Autodesk Inventor part; units mm, degrees
ref_plane "YZ Plane" through (0, 0, 0) normal (1, 0, 0) x (0, 1, 0)
ref_plane "XZ Plane" through (0, 0, 0) normal (0, 1, 0) x (-1, 0, 0)
ref_plane "XY Plane" through (0, 0, 0) normal (0, 0, 1) x (1, 0, 0)
sketch "Skizze1" plane through (0, 0, 0) normal (0, 0, 1) x (1, 0, 0)
  line L0 (-12.5, -12) -> (12.5, -12)
  line L1 (12.5, -12) -> (12.5, 12)
  line L2 (12.5, 12) -> (-12.5, 12)
  line L3 (-12.5, 12) -> (-12.5, -12)
  line L4 (-12.5, -12) -> (12.5, 12) construction
  line L5 (12.5, -12) -> (-12.5, 12) construction
  point P0 (0, 0)
  dimension "d0" = 25
  dimension "d1" = 24
extrude "Extrusion1" add sketch "Skizze1" along normal blind 1
sketch "Skizze2" plane through (0, 0, 1) normal (0, 0, 1) x (1, 0, 0)
  line L0 (-12.5, -12) -> (12.5, -12)
  line L1 (12.5, -12) -> (12.5, 12)
  line L2 (12.5, 12) -> (-12.5, 12)
  line L3 (-12.5, 12) -> (-12.5, -12)
  line L4 (12.5, 12) -> (-12.5, 12) construction
  line L5 (0, 12) -> (0, -12) construction
  line L6 (-12.5, -12) -> (12.5, -12) construction
  point P0 (0, 0)
  point P1 (-10.5, 10)
  point P2 (10.5, 10)
  point P3 (10.5, -3.5)
  point P4 (-10.5, -3.5)
  dimension "d4" = 2
  dimension "d5" = 2
  dimension "d6" = 8.5
  dimension "d7" = 2
hole "Bohrung1" at (-10.5, 10, 1) at (10.5, 10, 1) at (10.5, -3.5, 1) at (-10.5, -3.5, 1) direction (0, 0, -1) diameter 2.2 end through all
sketch "Skizze3" plane through (0, 0, 1) normal (0, 0, 1) x (1, 0, 0)
  circle A0 centre (10.5, -3.5) radius 1.1
  circle A1 centre (-10.5, 10) radius 1.1
  circle A2 centre (10.5, 10) radius 1.1
  circle A3 centre (-10.5, -3.5) radius 1.1
  line L0 (-12.5, -12) -> (12.5, -12)
  line L1 (12.5, -12) -> (12.5, 12)
  line L2 (12.5, 12) -> (-12.5, 12)
  line L3 (-12.5, 12) -> (-12.5, -12)
  line L4 (0, 12) -> (0, -12) construction
  point P0 (0, 0)
  point P1 (-9, 3)
  point P2 (9, 3)
  dimension "d16" = 9
  dimension "d17" = 18
hole "Bohrung2" at (-9, 3, 1) at (9, 3, 1) direction (0, 0, -1) diameter 1.82 end through all
properties part number "Waveshare Kamera PCB 24x25" material "Phenolharz"
Input: part model. Units: mm. Frame: model coordinates. Round coordinates to 2 decimals unless told otherwise and drop trailing zeros. Order: outer loops, then holes, each group sorted by start corner. A loop starts at its lowest first (then second) coordinate and runs counter-clockwise, first axis right, second up. Notation, with made-up numbers: (28, 25.5) - (65, 25.5) arc R30 ccw to (65, 56.5) - close; hole circle Ø7 at (69, -5). An arc over 180 degrees is marked (long way). Answer in a Markdown table with one row per item.
Item 1: Section query D-D (x = -10.5). Return the cut outline in (y, z).
Model answer:
| item | result |
|---|---|
| outline | (-12, 0) - (-4.6, 0) - (-4.6, 1) - (-12, 1) - close; (-2.4, 0) - (8.9, 0) - (8.9, 1) - (-2.4, 1) - close; (11.1, 0) - (12, 0) - (12, 1) - (11.1, 1) - close |
Item 2: Line query: line 1 (Y direction, x = -10.5, z = 0.55); line 2 (X direction, y = 10, z = 0.5); line 3 (X direction, y = -2.75, z = 0.7). Output: solid intervals per line, ascending.
Model answer:
| item | result |
|---|---|
| line 1 | y = -12 to -4.6, -2.4 to 8.9, 11.1 to 12 |
| line 2 | x = -12.5 to -11.6, -9.4 to 9.4, 11.6 to 12.5 |
| line 3 | x = -12.5 to -11.3, -9.7 to 9.7, 11.3 to 12.5 |
Item 3: Section query B-B (x = 9). Return the cut outline in (y, z).
Model answer:
| item | result |
|---|---|
| outline | (-12, 0) - (2.09, 0) - (2.09, 1) - (-12, 1) - close; (3.91, 0) - (12, 0) - (12, 1) - (3.91, 1) - close |
Item 4: Section query C-C (z = 0.8). Return the cut outline in (x, y).
Model answer:
| item | result |
|---|---|
| outline | (-12.5, -12) - (12.5, -12) - (12.5, 12) - (-12.5, 12) - close; hole circle Ø2.2 at (-10.5, -3.5); hole circle Ø2.2 at (-10.5, 10); hole circle Ø1.82 at (-9, 3); hole circle Ø1.82 at (9, 3); hole circle Ø2.2 at (10.5, -3.5); hole circle Ø2.2 at (10.5, 10) |
Item 5: Section query A-A (y = 3). Return the cut outline in (x, z).
Model answer:
| item | result |
|---|---|
| outline | (-12.5, 0) - (-9.91, 0) - (-9.91, 1) - (-12.5, 1) - close; (-8.09, 0) - (8.09, 0) - (8.09, 1) - (-8.09, 1) - close; (9.91, 0) - (12.5, 0) - (12.5, 1) - (9.91, 1) - close |
Item 6: Mould query, pull axis Y, two halves, no side actions, for faces 1 (the flat face through (0.2, 12, 0.5)), 2 (the flat face through (-0.2, -12, 0.5)), 3 (the cylindrical face through (10.921, 8.984, 0.493)). Classes: released by +Y, released by -Y, zero draft, split by the parting line, or undercut.
Model answer:
| item | result |
|---|---|
| face 1 | released by +Y |
| face 2 | released by -Y |
| face 3 | undercut |
Item 7: Pin query (flat end, axial travel): pin 1 (3.5 mm diameter, centred on x = -10.5, y = -3.5, fed in from -Z). Return the tip coordinate at first contact, or that it passes through.
Model answer:
| item | result |
|---|---|
| pin 1 | stops at z = 0 |
